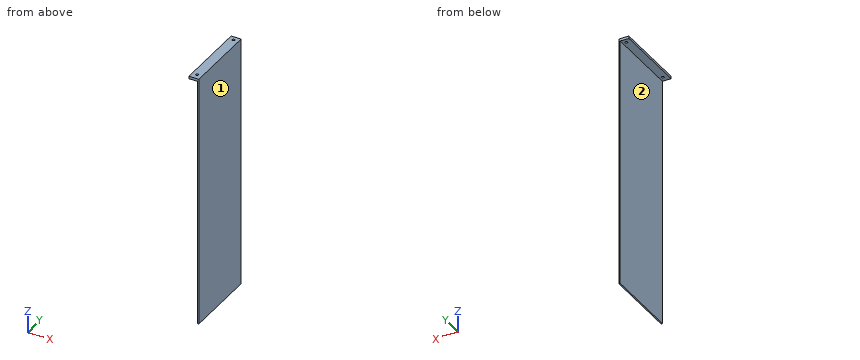
from build123d import *

# Parameters (mm, degrees)
F0_W     = 40
F0_H     = 300
F0_R     = 5
F1_DEPTH = 10
F2_W     = 5.453752
F2_H     = 300
F3_DEPTH = 1000


with BuildPart() as f1:
    # F0 (on Top) → F1 (new body)
    with BuildSketch(Plane.XY):
        Rectangle(F0_W, F0_H)
        with Locations((0, -126.960114)):
            Circle(F0_R, mode=Mode.SUBTRACT)
        with Locations((0, 131.599203)):
            Circle(F0_R, mode=Mode.SUBTRACT)
    extrude(amount=-F1_DEPTH)

    # F2 (on face) → F3 (join)
    with BuildSketch(Plane(origin=(0, 0, -10), x_dir=(1, 0, 0), z_dir=(0, 0, -1))):
        with Locations((17.273124, 0)):
            Rectangle(F2_W, F2_H)
    extrude(amount=F3_DEPTH)


solid = f1.part
Model file for the job. Use its own axes, mm. Face numbers are marked on the shaded views. A direction names the side the tool comes from. Give positions to 0.01 mm unless a question says otherwise; leave off trailing zeros. Order: outer loops, then holes, each group sorted by start corner. A loop starts at its lowest first (then second) coordinate and runs counter-clockwise, first axis right, second up. Notation, with made-up numbers: (4, -35.75) -> (42, -35.75) arc R19 ccw to (42, -18.75) -> close; hole circle Ø11 at (-24.5, -32). An arc over 180 degrees is marked (long way). Use CSV: the item, a comma, the result in double quotes.
1. 3-axis set-ups, long thin cutter, end or side, ignore diameter. For the marked faces 1 and 2: which of +Z, -Z, +X, -X, +Y, -Y reach the whole face in a straight line?
Outcome:
face 1,"+Z, -Z, +X, +Y, -Y"
face 2,"-Z, -X, +Y, -Y"
2. Drop flat-ended pins along their axis: pin 1 (12 mm diameter, centred on y = 16, z = -351, fed in from -X); pin 2 (12 mm diameter, centred on x = 3.5, y = -14, fed in from -Z). Give the stop position or say it passes through.
Outcome:
pin 1,"x = 14.55"
pin 2,"z = -10"
3. Band-saw the part on B-B, the plane z = -298.5. Give the cut face in (x, y).
Outcome:
outline,"(14.55, -150) -> (20, -150) -> (20, 150) -> (14.55, 150) -> close"
4. Band-saw the part on A-A, the plane y = 95. Give the cut face in (x, z).
Outcome:
outline,"(-20, -10) -> (14.55, -10) -> (14.55, -1010) -> (20, -1010) -> (20, 0) -> (-20, 0) -> close"
5. Drill centre lines: line 1 along Y through (x, z) = (0, -2); line 2 along X through (y, z) = (99.5, -566); line 3 along Z through (x, y) = (-11, 126). Where is each one in solid material? Low to high. Write a range as from..to.
Outcome:
line 1,"-150..-131.96, -121.96..126.6, 136.6..150"
line 2,"14.55..20"
line 3,"-10..0"
